Verification items for the finished model (mm, model axes). A direction names the side the tool comes from. Coordinates: 2 decimals unless noted, no trailing zeros. Loops run counter-clockwise (first coordinate to the right, second up) from the corner with the lowest first, then second, coordinate; pieces in that order, holes last. Notation, with made-up numbers: (-26, 0) -> (-18, 0) arc R33 cw to (-18, 36) -> close; hole circle Ø6 at (53.25, 17.25). An arc over 180 degrees is marked (long way). Use CSV: the item, a comma, the result in double quotes. Start each with the question number.
```python
from build123d import *

# Parameters (mm, degrees)
SALIENTE_EXTRUIR1_DEPTH = 10
CROQUIS2_R              = 1.25
CORTAR_EXTRUIR1_DEPTH   = 10
CROQUIS3_W              = 2
CROQUIS3_H              = 10
SALIENTE_EXTRUIR2_DEPTH = 2


with BuildPart() as part:
    # Croquis1 → Saliente-Extruir1 (new body)
    with BuildSketch(Plane(origin=(0, 0, 0), x_dir=(1, 0, 0), z_dir=(0, 1, 0))):
        Polygon((0, 0), (8, 0), (8, 4.5), (12.7, 4.5), (12.7, 0), (14.2, 0), (14.2, 6.5), (6, 6.5), (6, 2), (0, 2), align=None)
    extrude(amount=SALIENTE_EXTRUIR1_DEPTH)

    # Croquis2 → Cortar-Extruir1 (cut)
    with BuildSketch(Plane(origin=(0, 0, -2), x_dir=(-1, 0, 0), z_dir=(0, 0, -1))):
        with Locations((-3, 5)):
            Circle(CROQUIS2_R)
    extrude(amount=-CORTAR_EXTRUIR1_DEPTH, mode=Mode.SUBTRACT)

    # Croquis3 → Saliente-Extruir2 (add)
    with BuildSketch(Plane.ZY):
        with Locations((-1, 5)):
            Rectangle(CROQUIS3_W, CROQUIS3_H)
    extrude(amount=SALIENTE_EXTRUIR2_DEPTH)


solid = part.part
```
1. Cross-section at C-C, the plane z = -3. Record the boundary of the cut face in (x, y), plus the area to 3 significant figures.
2. Set-up check for faces 1 (the flat face through (1, 5, -2)), 2 (the flat face through (10, 5, -6.5)), 3 (the flat face through (12.7, 5, -2)): record each of +Z, -Z, +X, -X, +Y, -Y from which the full face is reachable in a straight line by a thin tool's end or side.
3. Cross-section at B-B, the plane y = 5. Record the boundary of the cut face in (x, z).
4. Release check for a two-part mould opening along X. For faces 4 (the flat face through (4, 6, 0)), 5 (the flat face through (10, 5, -4.5)), 6 (the flat face through (-2, 5, -1)) record: released by +X, released by -X, zero draft, split by the parting line, or undercut.
5. Cross-section at D-D, the plane x = 3. Record the boundary of the cut face in (y, z), plus the area to 3 significant figures.
6. Depth check by flat-ended pin: pin 1 (1.5 mm diameter, centred on y = 8.5, z = -2.5, fed in from -X); pin 2 (1 mm diameter, centred on x = 0, y = 2.5, fed in from -Z); pin 3 (1 mm diameter, centred on x = 11.5, y = 6.5, fed in from +Z). Enter the tip coordinate at first touch or a pass-through.
7. Cross-section at A-A, the plane z = -1.75. Record the boundary of the cut face in (x, y).
8. Scan lines: line 1 (Y direction, x = 3, z = -0.5); line 2 (X direction, y = 4.75, z = -2.5); line 3 (X direction, y = 8.25, z = -0.75). Record each from-to range of solid material in increasing order.
Solution:
1,outline,"(6, 0) -> (8, 0) -> (8, 10) -> (6, 10) -> close; (12.7, 0) -> (14.2, 0) -> (14.2, 10) -> (12.7, 10) -> close"
1,area,"35.0 mm2"
2,face 1,"-Z, -X, +Y, -Y"
2,face 2,"-Z, +X, -X, +Y, -Y"
2,face 3,"+Z, +Y, -Y"
3,outline,"(-2, -2) -> (1.75, -2) -> (1.75, 0) -> (-2, 0) -> close; (4.25, -2) -> (6, -2) -> (6, -6.5) -> (14.2, -6.5) -> (14.2, 0) -> (12.7, 0) -> (12.7, -4.5) -> (8, -4.5) -> (8, 0) -> (4.25, 0) -> close"
4,face 4,"zero draft"
4,face 5,"undercut"
4,face 6,"released by -X"
5,outline,"(0, -2) -> (3.75, -2) -> (3.75, 0) -> (0, 0) -> close; (6.25, -2) -> (10, -2) -> (10, 0) -> (6.25, 0) -> close"
5,area,"15.0 mm2"
6,pin 1,"stops at x = -2"
6,pin 2,"stops at z = -2"
6,pin 3,"stops at z = -4.5"
7,outline,"(-2, 0) -> (8, 0) -> (8, 10) -> (-2, 10) -> close; (12.7, 0) -> (14.2, 0) -> (14.2, 10) -> (12.7, 10) -> close; hole circle Ø2.5 at (3, 5)"
8,line 1,"y = 0 to 3.75, 6.25 to 10"
8,line 2,"x = 6 to 8, 12.7 to 14.2"
8,line 3,"x = -2 to 8, 12.7 to 14.2"
